Source: CAD feature listing. Evaluate the final solid. Frame: model axes, mm. Round coordinates to 2 decimals unless told otherwise and drop trailing zeros. Loops run counter-clockwise (first coordinate to the right, second up) from the corner with the lowest first, then second, coordinate; pieces in that order, holes last. Notation, with made-up numbers: (57.25, 55.25) - (87.25, 55.25) arc R17 cw to (87.25, 77.25) - close; hole circle Ø11 at (7.25, 19). An arc over 180 degrees is marked (long way). One line per question, with ' | ' between items.
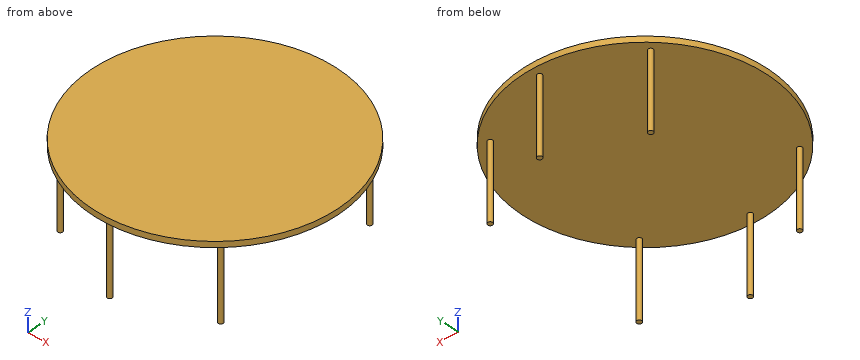
from build123d import *

# Parameters (mm, degrees)
SKETCH1_R      = 114.3
PLATFORM_DEPTH = 5.334
SKETCH3_R      = 2.286
PEGS_DEPTH     = 70.866


with BuildPart() as part:
    # Sketch1 → Platform (new body)
    with BuildSketch(Plane.XY):
        Circle(SKETCH1_R)
    extrude(amount=PLATFORM_DEPTH)

    # Sketch3 → Pegs (add)
    with BuildSketch(Plane(origin=(0, 0, 0), x_dir=(-1, 0, 0), z_dir=(0, 0, -1))):
        with Locations(Location((0, 105.41, 0), (0, 0, 180))):
            Circle(SKETCH3_R)
        with Locations(Location((-74.536125805, 74.536125805, 0), (0, 0, 180))):
            Circle(SKETCH3_R)
        with Locations(Location((-74.536125805, -74.536125805, 0), (0, 0, 180))):
            Circle(SKETCH3_R)
        with Locations(Location((0, -105.41, 0), (0, 0, 180))):
            Circle(SKETCH3_R)
        with Locations(Location((74.536125805, -74.536125805, 0), (0, 0, 180))):
            Circle(SKETCH3_R)
        with Locations(Location((74.536125805, 74.536125805, 0), (0, 0, 180))):
            Circle(SKETCH3_R)
    extrude(amount=PEGS_DEPTH)


solid = part.part
1. Section query A-A, the plane z = -38. Return loops of the section in (x, y).
Worked out:
outline: circle Ø4.57 at (-74.54, -74.54); circle Ø4.57 at (-74.54, 74.54); circle Ø4.57 at (0, -105.41); circle Ø4.57 at (0, 105.41); circle Ø4.57 at (74.54, -74.54); circle Ø4.57 at (74.54, 74.54)
2. Section query B-B, the plane y = 94.5. Return loops of the section in (x, z), plus the area to 3 significant figures.
Worked out:
outline: (-64.3, 0) - (64.3, 0) - (64.3, 5.33) - (-64.3, 5.33) - close | area: 686 mm2
3. Section query C-C, the plane x = -38. Return loops of the section in (y, z).
Worked out:
outline: (-107.8, 0) - (107.8, 0) - (107.8, 5.33) - (-107.8, 5.33) - close
4. Material intervals for probe 1 along Z at (x, y) = (-11, 68); probe 2 along X at (y, z) = (104, -26), sorted ascending.
Worked out:
probe 1: z = 0 to 5.33 | probe 2: x = -1.8 to 1.8
5. Contact query for a flat-ended pin moving along its axis: P1, Ø8, axis at x = -13, y = -37, coming from the -Z side. Output: stop coordinate, or through.
Worked out:
P1: stops at z = 0
